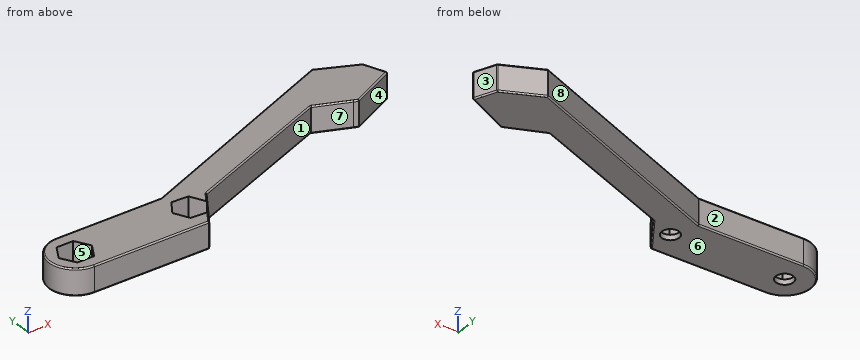
```python
from build123d import *

# Parameters (mm, degrees)
SKETCH1_R           = 1.65
BOSS_EXTRUDE1_DEPTH = 5
FILLET2_R           = 0.25
CUT_EXTRUDE1_DEPTH  = 4


with BuildPart() as part:
    # Sketch1 → Boss-Extrude1 (new body)
    # profile 1 of 2: a face of its own
    with BuildSketch(Plane.XY):
        with BuildLine():
            Line((-5.168635154, -1.464478016), (-25.218635154, -1.464478016))
            ThreePointArc((-25.218635154, -1.464478016), (-30.218635154, -6.464478016), (-25.218635154, -11.464478016))
            Line((-25.218635154, -11.464478016), (-3.218635154, -11.464478016))
            Line((-3.218635154, -11.464478016), (1.36555506, -4.468181425))
            ThreePointArc((1.36555506, -4.468181425), (-0.47833252, -2.282284635), (-3.218635154, -1.464478016))
            Line((-3.218635154, -1.464478016), (-5.168635154, -1.464478016))
        make_face()
        with Locations((-25.218635154, -6.464478016)):
            Circle(SKETCH1_R, mode=Mode.SUBTRACT)
        with Locations((-3.197929879, -6.257635448)):
            Circle(SKETCH1_R, mode=Mode.SUBTRACT)
    # profile 2 of 2: a face of its own
    with BuildSketch(Plane.XY):
        with BuildLine():
            Line((35.988446, 15.45724385), (-5.168635154, -1.464478016))
            Line((-5.168635154, -1.464478016), (-3.218635154, -1.464478016))
            ThreePointArc((-3.218635154, -1.464478016), (-0.47833252, -2.282284635), (1.36555506, -4.468181425))
            Line((1.36555506, -4.468181425), (29.450627286, 6.742809526))
            Line((29.450627286, 6.742809526), (35.767904523, 4.15974363))
            Line((35.767904523, 4.15974363), (36.572261964, 3.843716482))
            Line((36.572261964, 3.843716482), (45.016686804, 7.962377757))
            Line((45.016686804, 7.962377757), (43.305501447, 12.124329784))
            Line((43.305501447, 12.124329784), (35.988446, 15.45724385))
        make_face()
    extrude(amount=BOSS_EXTRUDE1_DEPTH)

    # Fillet2
    fillet2_edges = [part.edges().sort_by_distance(p)[0] for p in [
        (-14.218635154, -11.464478016, 0),
        (-30.218635154, -6.464478016, 0),
        (-15.193635154, -1.464478016, 0),
        (15.409905423, 6.996382917, 0),
        (-0.926540047, -7.966329721, 5),
        (39.646973723, 13.790786817, 0),
        (44.161094126, 10.04335377, 0),
        (40.794474384, 5.90304712, 0),
        (36.170083243, 4.001730056, 0),
        (32.609265904, 5.451276578, 0),
        (15.408091173, 1.137314051, 0),
        (-0.926540047, -7.966329721, 0),
        (15.408091173, 1.137314051, 5),
        (-3.218635154, -11.464478016, 2.5),
        (-5.168635154, -1.464478016, 2.5),
        (35.988446, 15.45724385, 2.5),
        (43.305501447, 12.124329784, 2.5),
        (45.016686804, 7.962377757, 2.5),
        (36.572261964, 3.843716482, 2.5),
        (35.767904523, 4.15974363, 2.5),
        (29.450627286, 6.742809526, 2.5),
        (1.36555506, -4.468181425, 2.5),
        (32.609265904, 5.451276578, 5),
        (36.170083243, 4.001730056, 5),
        (40.794474384, 5.90304712, 5),
        (44.161094126, 10.04335377, 5),
        (39.646973723, 13.790786817, 5),
        (15.409905423, 6.996382917, 5),
        (-15.193635154, -1.464478016, 5),
        (-30.218635154, -6.464478016, 5),
        (-14.218635154, -11.464478016, 5),
    ]]
    fillet(fillet2_edges, radius=FILLET2_R)

    # Sketch2 → Cut-Extrude1 (cut)
    with BuildSketch(Plane.XY.offset(5)):
        Polygon((-23.630921913, -9.214478016), (-22.043208673, -6.464478016), (-23.630921913, -3.714478016), (-26.806348394, -3.714478016), (-28.394061634, -6.464478016), (-26.806348394, -9.214478016), align=None)
        Polygon((-0.027560565, -6.436777135), (-1.45760397, -3.601585926), (-4.627973284, -3.422444239), (-6.368299193, -6.078493761), (-4.938255788, -8.91368497), (-1.767886474, -9.092826657), align=None)
    extrude(amount=-CUT_EXTRUDE1_DEPTH, mode=Mode.SUBTRACT)


solid = part.part
```
Could you check a few things on this model? Use its own coordinates, in mm. Face numbers are marked on the shaded views. A direction names the side the tool comes from. Round coordinates to 2 decimals unless told otherwise and drop trailing zeros. Write each loop counter-clockwise with the first axis right and the second up, starting at its lowest first coordinate (ties: lowest second). Pieces come first, ordered by that corner, then holes. Notation, with made-up numbers: M -14,-34.75 L 45,-34.75 A24 ccw 45,-22.75 Z; hole C 55.5,-12.75 d6. An arc over 180 degrees is marked long. Write each question's results on one line, items separated by ' | '. Start each with the question number.
1. I need wall thicknesses on L1, parallel to Y at x = -24.5, z = 4.05; L2, parallel to Y at x = -21, z = 0.85; L3, parallel to X at y = 11.5, z = 0.9. Which ranges of each line are inside material? Lowest first, please. Write a range as from..to.
2. Imagine slicing it at B-B on x = -8.5. List the corners of the cut face in (y, z) for me.
3. Thinking about a two-plate mould opening in X: for the marked faces 6, 7 and 8, which applies, +X half, -X half, draft (parallel to the pull), parting line (faces both ways), or undercut?
4. Imagine slicing it at A-A on z = 2.6. Count the separate pieces of the cut face and the enclosed holes in it, and give its area (3 significant figures).
5. On a 3-axis mill with a long thin cutter (end or side, diameter ignored), from which of +Z, -Z, +X, -X, +Y, -Y can I reach the whole of each face in a straight line? I mean the marked faces 1, 2, 3, 4 and 5. Say none if no direction works.
6. I'm going to push flat-ended pins straight in: pin 1 Ø2.5 at (x, y) = (-24, -5.5) entering from +Z; pin 2 Ø3 at (x, y) = (-3.5, -6.5) entering from +Z; pin 3 Ø2 at (x, z) = (-10, 1.5) entering from +Y; pin 4 Ø2 at (y, z) = (-4.5, 1.5) entering from -X. Where does each tip first touch, or does it pass through?
Result sheet:
1) L1: y = -11.46..-9.21, -3.71..-1.46 | L2: y = -11.46..-1.46 | L3: x = 26.36..43.56
2) outline: M -11.46,0.25 A0.25 ccw -11.21,0 L -1.71,0 A0.25 ccw -1.46,0.25 L -1.46,4.75 A0.25 ccw -1.71,5 L -11.21,5 A0.25 ccw -11.46,4.75 Z
3) face 6: draft | face 7: undercut | face 8: -X half
4) separate pieces: 1 | enclosed holes: 2 | area: 533 mm^2
5) face 1: +Z, -Z, -Y | face 2: +Z, -Z, -X, +Y | face 3: +Z, -Z, +X, +Y | face 4: +Z, -Z, +X, -Y | face 5: +Z
6) pin 1: stops at z = 5 | pin 2: stops at z = 1 | pin 3: stops at y = -1.46 | pin 4: stops at x = -30.12
